Read the model definition and answer for the solid it produces. Units are mm, in the model's axes. A direction names the side the tool comes from. Coordinates: 2 decimals unless noted, no trailing zeros. Write each loop counter-clockwise with the first axis right and the second up, starting at its lowest first coordinate (ties: lowest second). Pieces come first, ordered by that corner, then holes.
Item 1: Straight lines are drawn through the part: probe 1 along Z at (x, y) = (-14.5, 1.8); probe 2 along X at (y, z) = (0.2, 0.5); probe 3 along Y at (x, z) = (6.5, 0.5). For each, find the intervals that lie inside material, in ascending order.
Item 2: Section C-C (z = 7.75) is taken. Give the vertices of the cut face in (x, y).
Item 3: A tool of negligible diameter and unlimited length cuts with its end or side. For faces 4 (the face through (-12, 3, 0.6)), 5 (the face through (-6.25, 1, -1)), 6 (the face through (-12, 5, 5)), from which of +Z, -Z, +X, -X, +Y, -Y can it reach the whole face along a straight path? Write none if from no direction.
Item 4: Section A-A (x = -8.5) is taken. Give the vertices of the cut face in (y, z), then the cut area to 3 significant figures.
Item 5: Section D-D (y = 0.45) is taken. Give the vertices of the cut face in (x, z), then the cut area to 3 significant figures.
Item 6: Determine the mould class of faces 1 (the face through (-18.75, 2, -6)), 2 (the face through (-12, 2, -2.05)), 3 (the face through (-4, 2, -10)) for opening direction Z: released by +Z, released by -Z, zero draft, split by the parting line, or undercut.
Item 7: Section B-B (y = 3.7) is taken. Give the vertices of the cut face in (x, z).
Item 8: Each of these flat-tipped pins is pushed along its axis until it touches: P1, Ø0.8, axis at y = 1.5, z = -1, coming from the -X side; P2, Ø1.5, axis at y = 4, z = 1.5, coming from the +X side; P3, Ø2, axis at x = -7, z = 10, coming from the +Y side. Where does it stop, or does it pass through?
from build123d import *

# Parameters (mm, degrees)
SKETCH1_W           = 37.5
SKETCH1_H           = 40
BOSS_EXTRUDE1_DEPTH = 2.5
SKETCH2_W           = 12.5
SKETCH2_H           = 2.65
CUT_EXTRUDE1_DEPTH  = 28.528394432
SKETCH3_W           = 12.5
SKETCH3_H           = 17.95
SKETCH3_H_2         = 7.5
BOSS_EXTRUDE2_DEPTH = 2.5
SKETCH4_W           = 37.5
SKETCH4_H           = 10
CUT_EXTRUDE2_DEPTH  = 28.866871012


with BuildPart() as part:
    # Sketch1 → Boss-Extrude1 (new body)
    with BuildSketch(Plane(origin=(0, 0, 0), x_dir=(1, 0, 0), z_dir=(0, 1, 0))):
        Rectangle(SKETCH1_W, SKETCH1_H)
    extrude(amount=BOSS_EXTRUDE1_DEPTH)

    # Sketch2 → Cut-Extrude1 (cut, through all)
    with BuildSketch(Plane.XZ):
        with Locations((-12.5, -0.725)):
            Rectangle(SKETCH2_W, SKETCH2_H)
    extrude(amount=-CUT_EXTRUDE1_DEPTH, mode=Mode.SUBTRACT)

    # Sketch3 → Boss-Extrude2 (add)
    with BuildSketch(Plane(origin=(0, 2.5, 0), x_dir=(1, 0, 0), z_dir=(0, 1, 0))):
        with Locations((-12.5, 11.025)):
            Rectangle(SKETCH3_W, SKETCH3_H)
        with Locations((-12.5, -4.35)):
            Rectangle(SKETCH3_W, SKETCH3_H_2)
    extrude(amount=BOSS_EXTRUDE2_DEPTH)

    # Sketch4 → Cut-Extrude2 (cut, through all)
    with BuildSketch(Plane(origin=(0, 5, 0), x_dir=(1, 0, 0), z_dir=(0, 1, 0))):
        with Locations((0, 15)):
            Rectangle(SKETCH4_W, SKETCH4_H)
    extrude(amount=-CUT_EXTRUDE2_DEPTH, mode=Mode.SUBTRACT)

    # Chamfer1
    # the kernel refuses this chamfer: 5, 2.886751346 mm, written as the material it adds along each edge
    with BuildSketch(Plane(origin=(-6.25, 2.5, -2.05), x_dir=(0.9998132206222079, -0.019326765612700723, -1.5830863978385058e-15), z_dir=(0, 0, -1))) as chamfer1_piece_1_section:
        with BuildLine():
            Line((5.174171509, 0), (-0.230896973, -2.982845988))
            Line((-0.230896973, -2.982845988), (-0.330878295, -2.980913312))
            ThreePointArc((-0.330878295, -2.980913312), (-0.128843444, -1.491164065), (-0.099981322, 0.001932677))
            Line((-0.099981322, 0.001932677), (0.001932677, 0.099981322))
            ThreePointArc((0.001932677, 0.099981322), (2.588052093, 0.049990661), (5.176104186, 0.099981322))
            Line((5.176104186, 0.099981322), (5.174171509, 0))
        make_face()
    chamfer1_piece_1 = extrude(amount=7.95, mode=Mode.PRIVATE)
    chamfer1_piece_1 = split(chamfer1_piece_1, bisect_by=Plane(origin=(-6.25, 3.354735535, -6.025), z_dir=(1, 0, 0)), keep=Keep.TOP, mode=Mode.PRIVATE)
    chamfer1_piece_1 = split(chamfer1_piece_1, bisect_by=Plane(origin=(-4.46158964, 5, -6.025), z_dir=(0, -1, 0)), keep=Keep.TOP, mode=Mode.PRIVATE)
    add(chamfer1_piece_1)
    with BuildSketch(Plane(origin=(-6.25, 2.5, 8.1), x_dir=(0, -0.019326765612700723, 0.9998132206222079), z_dir=(-1, 0, 0))) as chamfer1_piece_2_section:
        with BuildLine():
            Line((5.174171509, 0), (-0.230896973, 2.982845988))
            Line((-0.230896973, 2.982845988), (-0.330878295, 2.980913312))
            ThreePointArc((-0.330878295, 2.980913312), (-0.128843444, 1.491164065), (-0.099981322, -0.001932677))
            Line((-0.099981322, -0.001932677), (0.001932677, -0.099981322))
            ThreePointArc((0.001932677, -0.099981322), (2.588052093, -0.049990661), (5.176104186, -0.099981322))
            Line((5.176104186, -0.099981322), (5.174171509, 0))
        make_face()
    chamfer1_piece_2 = extrude(amount=12.5, mode=Mode.PRIVATE)
    chamfer1_piece_2 = split(chamfer1_piece_2, bisect_by=Plane(origin=(-12.5, 5, 9.824344196), z_dir=(0, -1, 0)), keep=Keep.TOP, mode=Mode.PRIVATE)
    add(chamfer1_piece_2)
    with BuildSketch(Plane(origin=(-6.25, 2.5, 0.6), x_dir=(0.9998132206222079, -0.019326765612700723, 0), z_dir=(0, 0, 1))) as chamfer1_piece_3_section:
        with BuildLine():
            Line((5.174171509, 0), (-0.230896973, 2.982845988))
            Line((-0.230896973, 2.982845988), (-0.330878295, 2.980913312))
            ThreePointArc((-0.330878295, 2.980913312), (-0.128843444, 1.491164065), (-0.099981322, -0.001932677))
            Line((-0.099981322, -0.001932677), (0.001932677, -0.099981322))
            ThreePointArc((0.001932677, -0.099981322), (2.588052093, -0.049990661), (5.176104186, -0.099981322))
            Line((5.176104186, -0.099981322), (5.174171509, 0))
        make_face()
    chamfer1_piece_3 = extrude(amount=7.5, mode=Mode.PRIVATE)
    chamfer1_piece_3 = split(chamfer1_piece_3, bisect_by=Plane(origin=(-6.25, 3.354735535, 4.35), z_dir=(1, 0, 0)), keep=Keep.TOP, mode=Mode.PRIVATE)
    chamfer1_piece_3 = split(chamfer1_piece_3, bisect_by=Plane(origin=(-4.46158964, 5, 4.35), z_dir=(0, -1, 0)), keep=Keep.TOP, mode=Mode.PRIVATE)
    add(chamfer1_piece_3)
    with BuildSketch(Plane(origin=(-6.25, 2.5, 0.6), x_dir=(0.9998132206222079, -0.019326765612700723, 0), z_dir=(0, 0, 1))) as chamfer1_piece_4a_section:
        with BuildLine():
            Line((5.174171509, 0), (-0.230896973, 2.982845988))
            Line((-0.230896973, 2.982845988), (-0.330878295, 2.980913312))
            ThreePointArc((-0.330878295, 2.980913312), (-0.128843444, 1.491164065), (-0.099981322, -0.001932677))
            Line((-0.099981322, -0.001932677), (0.001932677, -0.099981322))
            ThreePointArc((0.001932677, -0.099981322), (2.588052093, -0.049990661), (5.176104186, -0.099981322))
            Line((5.176104186, -0.099981322), (5.174171509, 0))
        make_face()
    chamfer1_piece_4a = extrude(amount=20.435428773, mode=Mode.PRIVATE)
    chamfer1_piece_4a = split(chamfer1_piece_4a, bisect_by=Plane(origin=(-4.46158964, 3.354735535, 20), z_dir=(0, 0, -1)), keep=Keep.TOP, mode=Mode.PRIVATE)
    chamfer1_piece_4a = split(chamfer1_piece_4a, bisect_by=Plane(origin=(-6.25, 3.354735535, 14.05), z_dir=(1, 0, 0)), keep=Keep.TOP, mode=Mode.PRIVATE)
    chamfer1_piece_4a = split(chamfer1_piece_4a, bisect_by=Plane(origin=(-4.46158964, 5, 14.05), z_dir=(0, -1, 0)), keep=Keep.TOP, mode=Mode.PRIVATE)
    chamfer1_piece_4a = split(chamfer1_piece_4a, bisect_by=Plane(origin=(-4.46158964, 3.354735535, 8.1), z_dir=(0, 0, 1)), keep=Keep.TOP, mode=Mode.PRIVATE)
    with BuildSketch(Plane(origin=(6.685428773, 2.5, 8.1), x_dir=(0, -0.019326765612700723, 0.9998132206222079), z_dir=(-1, 0, 0))) as chamfer1_piece_4b_section:
        with BuildLine():
            Line((5.174171509, 0), (-0.230896973, 2.982845988))
            Line((-0.230896973, 2.982845988), (-0.330878295, 2.980913312))
            ThreePointArc((-0.330878295, 2.980913312), (-0.128843444, 1.491164065), (-0.099981322, -0.001932677))
            Line((-0.099981322, -0.001932677), (0.001932677, -0.099981322))
            ThreePointArc((0.001932677, -0.099981322), (2.588052093, -0.049990661), (5.176104186, -0.099981322))
            Line((5.176104186, -0.099981322), (5.174171509, 0))
        make_face()
    chamfer1_piece_4b = extrude(amount=25.435428773, mode=Mode.PRIVATE)
    chamfer1_piece_4b = split(chamfer1_piece_4b, bisect_by=Plane(origin=(0.217714387, 5, 9.824344196), z_dir=(0, -1, 0)), keep=Keep.TOP, mode=Mode.PRIVATE)
    chamfer1_piece_4b = split(chamfer1_piece_4b, bisect_by=Plane(origin=(-6.25, 3.374002547, 9.824344196), z_dir=(1, 0, 0)), keep=Keep.TOP, mode=Mode.PRIVATE)
    chamfer1_piece_4 = chamfer1_piece_4a & chamfer1_piece_4b
    add(chamfer1_piece_4)


solid = part.part
Established:
1. probe 1: z = -10 to -2.05, 0.6 to 20
1. probe 2: x = -6.25 to 18.75
1. probe 3: y = 0 to 2.5
2. outline: (-18.75, 0) - (18.75, 0) - (18.75, 2.5) - (-1.25, 2.5) - (-5.58, 5) - (-18.75, 5) - close
3. face 4: -X, +Y
3. face 5: -X, +Y, -Y
3. face 6: +Z, -Z, +X, -X, +Y
4. outline: (0, -10) - (5, -10) - (5, -2.05) - (0, -2.05) - close; (0, 0.6) - (5, 0.6) - (5, 8.77) - (2.5, 13.1) - (2.5, 20) - (0, 20) - close
4. area: 114 mm2
5. outline: (-18.75, -10) - (18.75, -10) - (18.75, 20) - (-18.75, 20) - (-18.75, 0.6) - (-6.25, 0.6) - (-6.25, -2.05) - (-18.75, -2.05) - close
5. area: 1,090 mm2
6. face 1: zero draft
6. face 2: undercut
6. face 3: released by -Z
7. outline: (-18.75, -10) - (-3.33, -10) - (-3.33, -2.05) - (-18.75, -2.05) - close; (-18.75, 0.6) - (-3.33, 0.6) - (-3.33, 11.02) - (-18.75, 11.02) - close
8. P1: stops at x = -6.25
8. P2: stops at x = -2.55
8. P3: stops at y = 4.87
